from build123d import *

# Parameters (mm, degrees)
SKETCH1_R               = 16.485
SKETCH1_R_2             = 14.235
BOSS_EXTRUDE1_DEPTH     = 63
SKETCH2_R               = 4.125
CUT_EXTRUDE1_DEPTH      = 73.991616813
CUT_EXTRUDE2_START      = -32.970000348
CUT_EXTRUDE2_DEPTH      = 32.970000348
CUT_EXTRUDE4_DEPTH      = 68.175222223
CUT_EXTRUDE4_DEPTH_BACK = 15
BOSS_EXTRUDE2_DEPTH     = 0.875
SKETCH9_W               = 2.280579787
SKETCH9_H               = 1.75
BOSS_EXTRUDE4_DEPTH     = 7.5
SKETCH10_W              = 0.221248718
SKETCH10_H              = 10
CUT_EXTRUDE5_DEPTH      = 2.5
BOSS_EXTRUDE5_REACH     = 77.139
SKETCH11_R              = 7.75
SKETCH11_R_2            = 4.125
CUT_EXTRUDE7_DEPTH      = 10


# Read off the part's stored shape, not the designer's step: Cut-Extrude2
with BuildPart() as part:
    # Sketch1 → Boss-Extrude1 (new body)
    with BuildSketch(Plane(origin=(0, 0, 0), x_dir=(1, 0, 0), z_dir=(0, 1, 0))):
        with Locations(Location((0, 0, 0), (0, 0, 270))):
            Circle(SKETCH1_R)
        with Locations(Location((0, 0, 0), (0, 0, 270))):
            Circle(SKETCH1_R_2, mode=Mode.SUBTRACT)
    extrude(amount=BOSS_EXTRUDE1_DEPTH)

    # Sketch2 → Cut-Extrude1 (cut, through all)
    with BuildSketch(Plane(origin=(16.485, 0, 0), x_dir=(0, 0, -1), z_dir=(1, 0, 0))):
        with Locations((0, 7.75)):
            Circle(SKETCH2_R)
    extrude(amount=-CUT_EXTRUDE1_DEPTH, mode=Mode.SUBTRACT)

    # Cut-Extrude2 outline → Cut-Extrude2 (cut)
    with BuildSketch(Plane(origin=(16.485, 0, 0), x_dir=(0, 0, -1), z_dir=(1, 0, 0)).offset(CUT_EXTRUDE2_START)):
        Polygon((5.5, 63), (-16.485, 63), (-16.485, 61.04), (-2.5, 61.04), (5.5, 61.54), align=None)
        with BuildLine():
            Line((-2.5, 59.29), (-16.485, 59.29))
            Line((-16.485, 59.29), (-16.485, 0))
            Line((-16.485, 0), (1.7e-08, 0))
            ThreePointArc((1.7e-08, 0), (-7.75, 7.749999991), (0, 15.5))
            Line((0, 15.5), (5.5, 35.5))
            Line((5.5, 35.5), (5.5, 58.79))
            Line((5.5, 58.79), (-2.5, 59.29))
        make_face()
        with BuildLine():
            ThreePointArc((7.75, 7.75), (5.48007756, 2.269922452), (1.7e-08, 0))
            Line((1.7e-08, 0), (16.485, 0))
            Line((16.485, 0), (16.485, 59.29))
            Line((16.485, 59.29), (7.75, 7.75))
        make_face()
    extrude(amount=CUT_EXTRUDE2_DEPTH, mode=Mode.SUBTRACT)

    # Sketch6 → Cut-Extrude4 (cut, two sides: drawn at the far end of the back side and taken through both)
    with BuildSketch(Plane(origin=(0, 63, 0), x_dir=(1, 0, 0), z_dir=(0, 1, 0)).offset(-CUT_EXTRUDE4_DEPTH_BACK)):
        Polygon((-103.23133718, 5.5), (-15.540438379, 5.5), (-13.1295554, 5.5), (0, 0), (14.013751282, -2.5), (16.294331069, -2.5), (103.985229871, -2.5), (97.219313689, -177.751240534), (-109.997253363, -169.751240534), align=None)
    extrude(amount=CUT_EXTRUDE4_DEPTH + CUT_EXTRUDE4_DEPTH_BACK, mode=Mode.SUBTRACT)

    # Sketch7 → Boss-Extrude2 (add, symmetric)
    with BuildSketch(Plane(origin=(0, 60.165, 0), x_dir=(1, 0, 0), z_dir=(0, 1, 0))):
        with BuildLine():
            ThreePointArc((0.300302569, 16.48226451), (10.624070386, 12.604933694), (16.193433276, 3.086736743))
            Line((16.193433276, 3.086736743), (16.127170788, 6.755707763))
            ThreePointArc((16.127170788, 6.755707763), (12.065849771, 12.654662947), (5.980222206, 16.430525474))
            Line((5.980222206, 16.430525474), (0.300302569, 16.48226451))
        make_face()
    extrude(amount=BOSS_EXTRUDE2_DEPTH, both=True)

    # Sketch9 → Boss-Extrude4 (add)
    with BuildSketch(Plane.XY.offset(2.5)):
        with Locations((15.154041176, 60.165)):
            Rectangle(SKETCH9_W, SKETCH9_H)
    extrude(amount=BOSS_EXTRUDE4_DEPTH)

    # Sketch10 → Cut-Extrude5 (cut, symmetric)
    with BuildSketch(Plane(origin=(0, 61.04, 0), x_dir=(1, 0, 0), z_dir=(0, 1, 0))):
        with Locations((14.124375641, -5)):
            Rectangle(SKETCH10_W, SKETCH10_H)
    extrude(amount=CUT_EXTRUDE5_DEPTH, both=True, mode=Mode.SUBTRACT)

    # Sketch11 → Boss-Extrude5 (add, up to next)
    with BuildSketch(Plane(origin=(21, 0, 0), x_dir=(0, 0, -1), z_dir=(1, 0, 0)), mode=Mode.PRIVATE) as boss_extrude5_sk1:
        with Locations((0, 7.75)):
            Circle(SKETCH11_R)
        with Locations((0, 7.75)):
            Circle(SKETCH11_R_2, mode=Mode.SUBTRACT)
    boss_extrude5_tool1 = extrude(boss_extrude5_sk1.sketch, amount=-BOSS_EXTRUDE5_REACH, mode=Mode.PRIVATE) - part.part
    add(boss_extrude5_tool1.solids().sort_by_distance((21, 7.75, 7.530797))[0])

    # Sketch16 → Cut-Extrude7 (cut)
    with BuildSketch(Plane(origin=(0, 63, 0), x_dir=(1, 0, 0), z_dir=(0, 1, 0))):
        Polygon((16.127170788, 6.755707763), (16.294331069, -2.5), (18.305732321, -2.5), (18.305732321, 6.795053101), align=None)
    extrude(amount=-CUT_EXTRUDE7_DEPTH, mode=Mode.SUBTRACT)


solid = part.part
Geometry: final body of the model. Coordinates: model frame, mm. A direction names the side the tool comes from. Coordinates: 2 decimals unless noted, no trailing zeros. Order: outer loops, then holes, each group sorted by start corner. A loop starts at its lowest first (then second) coordinate and runs counter-clockwise, first axis right, second up.
1) First-contact query: P1, Ø6, axis at y = 17.5, z = -10, coming from the +X side (3 decimals); P2, Ø2.5, axis at x = 15, z = 8, coming from the +Y side; P3, Ø0.7, axis at x = 15, y = 62, coming from the +Z side; P4, Ø7.5, axis at y = 7.75, z = 0, coming from the -X side. Flat tips, straight axial feed; report the tip coordinate or a pass-through.
Result sheet:
P1: stops at x = 14.925
P2: stops at y = 61.04
P3: stops at z = -5.5
P4: passes through
2) Section A-A (y = 32.5). Return loops of the section in (x, z) (3 decimals).
Result sheet:
outline: (-15.808, -4.675) arc R16.485 ccw to (-11.361, -11.945) - (-7.743, -11.945) arc R14.235 cw to (-13.445, -4.675) - close; (7.743, -11.945) - (11.361, -11.945) arc R16.485 ccw to (15.808, -4.675) - (13.445, -4.675) arc R14.235 cw to start
3) Section D-D (z = -8.5). Return loops of the section in (x, y), then the cut area to 3 significant figures.
Result sheet:
outline: (-14.12, 12.18) - (-11.42, 12.18) - (-11.42, 63) - (-14.12, 63) - close; (11.42, 12.18) - (14.12, 12.18) - (14.12, 59.29) - (15.28, 59.29) - (15.28, 61.04) - (14.12, 61.04) - (14.12, 63) - (11.42, 63) - close
area: 277 mm2
4) Set-up query: faces 1 (the flat face through (11.2, 61.04, -12.3)), 2 (the flat face through (16.294, 60, 6)), 3 (the flat face through (11.2, 59.29, -12.3)), 4 (the flat face through (15, 61.04, 6)), 5 (the flat face through (15.16, 25.36, -2.71)). Return all of +Z, -Z, +X, -X, +Y, -Y with unobstructed straight access to the full face (end or side cutting, diameter ignored); none if empty.
Result sheet:
face 1: -Z, +X, +Y
face 2: +Z, -Z, +X, +Y
face 3: -Z, +X
face 4: +Z, +X, -X, +Y
face 5: +Z, +X, -X
5) Draft query along Y for faces 6 (the flat face through (14, 62, -5.5)), 7 (the flat face through (15.041, 61.286, -1.444)), 8 (the flat face through (15, 59.29, 6)). Return one class per face: released by +Y, released by -Y, zero draft, split by the parting line, or undercut.
Result sheet:
face 6: zero draft
face 7: released by +Y
face 8: undercut
6) Section C-C (x = 8). Return loops of the section in (y, z).
Result sheet:
outline: (31.5, -11.77) - (47.07, -14.41) - (59.29, -14.41) - (59.29, -15.55) - (61.04, -15.55) - (61.04, -14.41) - (63, -14.41) - (63, -11.77) - close
7) Ray query, probe 1 along Z at (x, y) = (14.35, 7.75) (3 decimals); probe 2 along Y at (x, z) = (17.35, 0) (3 decimals); probe 3 along X at (y, z) = (58, -11.25). Return the intervals inside material, ascending.
Result sheet:
probe 1: z = -7.75 to -4.125, 4.125 to 7.75
probe 2: y = 0 to 3.625, 11.875 to 15.5
probe 3: x = -12.05 to -8.72, 8.72 to 12.05
8) Section B-B (z = 6.5). Return loops of the section in (x, y) (3 decimals).
Result sheet:
outline: (-15.149, 3.53) - (-12.664, 3.53) - (-12.664, 11.97) - (-15.149, 11.97) - close; (12.664, 3.53) - (21, 3.53) - (21, 11.97) - (12.664, 11.97) - close; (14.235, 59.29) - (16.294, 59.29) - (16.294, 61.04) - (14.235, 61.04) - close
